```python
from build123d import *

# Parameters (mm, degrees)
SKETCH_1_R               = 17.4
EXTRUDE_1_DEPTH          = 5.6
SKETCH_2_R               = 1.7
CUT_EXTRUDE_1_DEPTH      = 26.23648153
SKETCH_3_R               = 7
CUT_EXTRUDE_2_DEPTH      = 26.23648153
SKETCH_4_R               = 2.8
CUT_EXTRUDE_3_DEPTH      = 3
SKETCH_5_R               = 1.7
CUT_EXTRUDE_4_DEPTH      = 26.23648153
CUT_EXTRUDE_5_DEPTH      = 2.5
SKETCH_7_W               = 16.1
SKETCH_7_H               = 16.1
CUT_EXTRUDE_6_DEPTH      = 1.5
CHAMFER_1_SIZE           = 0.5
SKETCH_9_W               = 2.2
SKETCH_9_H               = 8
SKETCH_9_W_2             = 8
SKETCH_9_H_2             = 2.2
CUT_EXTRUDE_7_DEPTH      = 26.281613873
BOSS_EXTRUDE1_DEPTH      = 5.6
BOSS_EXTRUDE1_DEPTH_BACK = 4
SKETCH1_R                = 20.65
SKETCH1_R_2              = 17.4
SKETCH3_R                = 23
SKETCH3_R_2              = 20.65
BOSS_EXTRUDE2_DEPTH      = 2.5
SKETCH4_R                = 18
CUT_EXTRUDE3_DEPTH       = 4
SKETCH5_W                = 1
SKETCH5_H                = 8
CUT_EXTRUDE4_DEPTH       = 10
CUT_EXTRUDE6_DEPTH       = 10
FILLET3_R                = 1
SKETCH9_R                = 23
CUT_EXTRUDE8_DEPTH       = 6.5


with BuildPart() as part:
    # 草图1 → 凸台-拉伸1 (new body)
    with BuildSketch(Plane.XY):
        Circle(SKETCH_1_R)
    extrude(amount=EXTRUDE_1_DEPTH)

    # 草图2 → 切除-拉伸1 (cut, through all)
    with BuildSketch(Plane.XY.offset(5.6)):
        with Locations((-6.717514421, 6.717514421)):
            Circle(SKETCH_2_R)
        with Locations((6.717514421, -6.717514421)):
            Circle(SKETCH_2_R)
    extrude(amount=-CUT_EXTRUDE_1_DEPTH, mode=Mode.SUBTRACT)

    # 草图3 → 切除-拉伸2 (cut, through all)
    with BuildSketch(Plane.XY.offset(5.6)):
        Circle(SKETCH_3_R)
    extrude(amount=-CUT_EXTRUDE_2_DEPTH, mode=Mode.SUBTRACT)

    # 草图4 → 切除-拉伸3 (cut)
    with BuildSketch(Plane.XY.offset(5.6)):
        with Locations((-6.717514421, 6.717514421)):
            Circle(SKETCH_4_R)
        with Locations((6.717514421, -6.717514421)):
            Circle(SKETCH_4_R)
    extrude(amount=-CUT_EXTRUDE_3_DEPTH, mode=Mode.SUBTRACT)

    # 草图5 → 切除-拉伸4 (cut, through all)
    with BuildSketch(Plane.XY.offset(5.6)):
        with Locations((8.05, 8)):
            Circle(SKETCH_5_R)
        with Locations((-8.05, -8)):
            Circle(SKETCH_5_R)
    extrude(amount=-CUT_EXTRUDE_4_DEPTH, mode=Mode.SUBTRACT)

    # 草图6 → 切除-拉伸5 (cut)
    with BuildSketch(Plane(origin=(0, 0, 0), x_dir=(-1, 0, 0), z_dir=(0, 0, -1))):
        Polygon((4.766838493, -8), (6.408419246, -10.84330127), (9.691580754, -10.84330127), (11.333161507, -8), (9.691580754, -5.15669873), (6.408419246, -5.15669873), align=None)
        Polygon((-4.766838493, 8), (-6.408419246, 10.84330127), (-9.691580754, 10.84330127), (-11.333161507, 8), (-9.691580754, 5.15669873), (-6.408419246, 5.15669873), align=None)
    extrude(amount=-CUT_EXTRUDE_5_DEPTH, mode=Mode.SUBTRACT)

    # 草图7 → 切除-拉伸6 (cut)
    with BuildSketch(Plane.XY.offset(5.6)):
        Rectangle(SKETCH_7_W, SKETCH_7_H)
    extrude(amount=-CUT_EXTRUDE_6_DEPTH, mode=Mode.SUBTRACT)

    # 倒角1
    chamfer_1_edges = [part.edges().sort_by_distance(p)[0] for p in [
        (8.05, 1.022551258, 5.6),
        (1.047918985, 8.05, 5.6),
        (-8.05, -1.022551258, 5.6),
        (-1.047918985, -8.05, 5.6),
    ]]
    chamfer(chamfer_1_edges, length=CHAMFER_1_SIZE)

    # 草图8 → 旋转1 (revolve)
    with BuildSketch(Plane(origin=(0, 0, 0), x_dir=(0, 0, -1), z_dir=(1, 0, 0)), mode=Mode.PRIVATE) as revolve_1_sk:
        Polygon((0, 17.4), (0, 17.2), (0.2, 17.4), align=None)
    revolve(revolve_1_sk.sketch.rotate(Axis((0, 0, 0), (0, 0, 1)), 90), axis=Axis((0, 0, 0), (0, 0, 1)))

    # 草图9 → 切除-拉伸7 (cut, through all)
    with BuildSketch(Plane.XY.offset(5.6)):
        with Locations((14.6, 0)):
            Rectangle(SKETCH_9_W, SKETCH_9_H)
        with Locations((0, 14.6)):
            Rectangle(SKETCH_9_W_2, SKETCH_9_H_2)
        with Locations((-14.6, 0)):
            Rectangle(SKETCH_9_W, SKETCH_9_H)
        with Locations((0, -14.6)):
            Rectangle(SKETCH_9_W_2, SKETCH_9_H_2)
    extrude(amount=-CUT_EXTRUDE_7_DEPTH, mode=Mode.SUBTRACT)

    # Sketch1 → Boss-Extrude1 (add, two sides: drawn at the far end of the back side and taken through both)
    with BuildSketch(Plane.XY.offset(-BOSS_EXTRUDE1_DEPTH_BACK)):
        Circle(SKETCH1_R)
        Circle(SKETCH1_R_2, mode=Mode.SUBTRACT)
    extrude(amount=BOSS_EXTRUDE1_DEPTH + BOSS_EXTRUDE1_DEPTH_BACK)

    # Sketch3 → Boss-Extrude2 (add)
    with BuildSketch(Plane(origin=(0, 0, -4), x_dir=(-1, 0, 0), z_dir=(0, 0, -1))):
        Circle(SKETCH3_R)
        with Locations(Location((0, 0, 0), (0, 0, 180))):
            Circle(SKETCH3_R_2, mode=Mode.SUBTRACT)
    extrude(amount=-BOSS_EXTRUDE2_DEPTH)

    # Sketch4 → Cut-Extrude3 (cut)
    with BuildSketch(Plane(origin=(0, 0, -4), x_dir=(-1, 0, 0), z_dir=(0, 0, -1))):
        Circle(SKETCH4_R)
    extrude(amount=-CUT_EXTRUDE3_DEPTH, mode=Mode.SUBTRACT)

    # Sketch5 → Cut-Extrude4 (cut)
    with BuildSketch(Plane(origin=(0, 0, -4), x_dir=(-1, 0, 0), z_dir=(0, 0, -1))):
        with Locations((22.5, 0)):
            Rectangle(SKETCH5_W, SKETCH5_H)
        with Locations((-22.5, 0)):
            Rectangle(SKETCH5_W, SKETCH5_H)
    extrude(amount=-CUT_EXTRUDE4_DEPTH, mode=Mode.SUBTRACT)

    # Sketch7 → Cut-Extrude6 (cut)
    with BuildSketch(Plane(origin=(0, 0, -4), x_dir=(-1, 0, 0), z_dir=(0, 0, -1))):
        with BuildLine():
            Line((0, 18), (0, 22.3))
            Line((0, 22.3), (-2.6, 22.3))
            Line((-2.6, 22.3), (-2.6, 17.811232411))
            ThreePointArc((-2.6, 17.811232411), (-1.303421766, 17.952746077), (0, 18))
        make_face()
        with BuildLine():
            Line((0, 17.5), (0, 18))
            ThreePointArc((0, 18), (-1.303421766, 17.952746077), (-2.6, 17.811232411))
            Line((-2.6, 17.811232411), (-2.6, 17.5))
            Line((-2.6, 17.5), (0, 17.5))
        make_face()
        with BuildLine():
            Line((2.6, 22.3), (0, 22.3))
            Line((0, 22.3), (0, 18))
            ThreePointArc((0, 18), (1.303421766, 17.952746077), (2.6, 17.811232411))
            Line((2.6, 17.811232411), (2.6, 22.3))
        make_face()
        with BuildLine():
            ThreePointArc((2.6, 17.811232411), (1.303421766, 17.952746077), (0, 18))
            Line((0, 18), (0, 17.5))
            Line((0, 17.5), (2.6, 17.5))
            Line((2.6, 17.5), (2.6, 17.811232411))
        make_face()
    extrude(amount=-CUT_EXTRUDE6_DEPTH, mode=Mode.SUBTRACT)

    # Fillet3
    # the kernel refuses this fillet: 1 mm, written as the material it adds along each edge
    with BuildSketch(Plane(origin=(2.6, 22.3, -4), x_dir=(-1, 0, 0), z_dir=(0, 0, 1))) as fillet3_piece_1:
        with BuildLine():
            CenterArc((FILLET3_R, FILLET3_R), FILLET3_R, 180, 90)
            Line((0, FILLET3_R), (-FILLET3_R * 0.02, FILLET3_R))
            Line((-FILLET3_R * 0.02, FILLET3_R), (-FILLET3_R * 0.02, -FILLET3_R * 0.02))
            Line((-FILLET3_R * 0.02, -FILLET3_R * 0.02), (FILLET3_R, -FILLET3_R * 0.02))
            Line((FILLET3_R, -FILLET3_R * 0.02), (FILLET3_R, 0))
        make_face()
    extrude(amount=2.5)
    with BuildSketch(Plane(origin=(-2.6, 22.3, -4), x_dir=(1, 0, 0), z_dir=(0, 0, 1))) as fillet3_piece_2:
        with BuildLine():
            CenterArc((FILLET3_R, -FILLET3_R), FILLET3_R, 90, 90)
            Line((0, -FILLET3_R), (-FILLET3_R * 0.02, -FILLET3_R))
            Line((-FILLET3_R * 0.02, -FILLET3_R), (-FILLET3_R * 0.02, FILLET3_R * 0.02))
            Line((-FILLET3_R * 0.02, FILLET3_R * 0.02), (FILLET3_R, FILLET3_R * 0.02))
            Line((FILLET3_R, FILLET3_R * 0.02), (FILLET3_R, 0))
        make_face()
    extrude(amount=2.5)
    with BuildSketch(Plane(origin=(-2.6, 17.5, -6), x_dir=(0, 1, 0), z_dir=(0, 0, 1))) as fillet3_piece_3_section:
        with BuildLine():
            CenterArc((FILLET3_R, -FILLET3_R), FILLET3_R, 90, 90)
            Line((0, -FILLET3_R), (-FILLET3_R * 0.02, -FILLET3_R))
            Line((-FILLET3_R * 0.02, -FILLET3_R), (-FILLET3_R * 0.02, FILLET3_R * 0.02))
            Line((-FILLET3_R * 0.02, FILLET3_R * 0.02), (FILLET3_R, FILLET3_R * 0.02))
            Line((FILLET3_R, FILLET3_R * 0.02), (FILLET3_R, 0))
        make_face()
    fillet3_piece_3 = extrude(amount=11.6, mode=Mode.PRIVATE)
    fillet3_piece_3 = split(fillet3_piece_3, bisect_by=Plane(origin=(-2.544482942, 18.024809788, 0), z_dir=(0, 0, -1)), keep=Keep.TOP, mode=Mode.PRIVATE)
    fillet3_piece_3 = fillet3_piece_3 - Plane(origin=(0, 0, -2), x_dir=(-1, 0, 0), z_dir=(0, 0, -1)) * Cylinder(18, 28, mode=Mode.PRIVATE)
    fillet3_piece_3 = split(fillet3_piece_3, bisect_by=Plane(origin=(-2.544482942, 18.024809788, -4), z_dir=(0, 0, 1)), keep=Keep.TOP, mode=Mode.PRIVATE)
    add(fillet3_piece_3)
    with BuildSketch(Plane(origin=(-2.6, 17.5, 0), x_dir=(0, 1, 0), z_dir=(0, 0, 1))) as fillet3_piece_4_section:
        with BuildLine():
            CenterArc((FILLET3_R, -FILLET3_R), FILLET3_R, 90, 90)
            Line((0, -FILLET3_R), (-FILLET3_R * 0.02, -FILLET3_R))
            Line((-FILLET3_R * 0.02, -FILLET3_R), (-FILLET3_R * 0.02, FILLET3_R * 0.02))
            Line((-FILLET3_R * 0.02, FILLET3_R * 0.02), (FILLET3_R, FILLET3_R * 0.02))
            Line((FILLET3_R, FILLET3_R * 0.02), (FILLET3_R, 0))
        make_face()
    fillet3_piece_4 = extrude(amount=5.6, mode=Mode.PRIVATE)
    fillet3_piece_4 = fillet3_piece_4 - Plane(origin=(0, 0, 2.8), x_dir=(-1, 0, 0), z_dir=(0, 0, -1)) * Cylinder(18, 16, mode=Mode.PRIVATE)
    add(fillet3_piece_4)
    with BuildSketch(Plane(origin=(-2.6, 17.5, 0), x_dir=(0, 1, 0), z_dir=(0, 0, 1))) as fillet3_piece_5_section:
        with BuildLine():
            CenterArc((FILLET3_R, -FILLET3_R), FILLET3_R, 90, 90)
            Line((0, -FILLET3_R), (-FILLET3_R * 0.02, -FILLET3_R))
            Line((-FILLET3_R * 0.02, -FILLET3_R), (-FILLET3_R * 0.02, FILLET3_R * 0.02))
            Line((-FILLET3_R * 0.02, FILLET3_R * 0.02), (FILLET3_R, FILLET3_R * 0.02))
            Line((FILLET3_R, FILLET3_R * 0.02), (FILLET3_R, 0))
        make_face()
    fillet3_piece_5 = extrude(amount=5.6, mode=Mode.PRIVATE)
    fillet3_piece_5 = fillet3_piece_5 & Plane(origin=(0, 0, 2.8), x_dir=(-1, 0, 0), z_dir=(0, 0, -1)) * Cylinder(18, 16, mode=Mode.PRIVATE)
    add(fillet3_piece_5)
    with BuildSketch(Plane(origin=(2.6, 17.5, -6), x_dir=(-1, 0, 0), z_dir=(0, 0, 1))) as fillet3_piece_6_section:
        with BuildLine():
            CenterArc((FILLET3_R, -FILLET3_R), FILLET3_R, 90, 90)
            Line((0, -FILLET3_R), (-FILLET3_R * 0.02, -FILLET3_R))
            Line((-FILLET3_R * 0.02, -FILLET3_R), (-FILLET3_R * 0.02, FILLET3_R * 0.02))
            Line((-FILLET3_R * 0.02, FILLET3_R * 0.02), (FILLET3_R, FILLET3_R * 0.02))
            Line((FILLET3_R, FILLET3_R * 0.02), (FILLET3_R, 0))
        make_face()
    fillet3_piece_6 = extrude(amount=11.6, mode=Mode.PRIVATE)
    fillet3_piece_6 = split(fillet3_piece_6, bisect_by=Plane(origin=(2.544482942, 18.024809788, 0), z_dir=(0, 0, -1)), keep=Keep.TOP, mode=Mode.PRIVATE)
    fillet3_piece_6 = fillet3_piece_6 - Plane(origin=(0, 0, -2), x_dir=(-1, 0, 0), z_dir=(0, 0, -1)) * Cylinder(18, 28, mode=Mode.PRIVATE)
    fillet3_piece_6 = split(fillet3_piece_6, bisect_by=Plane(origin=(2.544482942, 18.024809788, -4), z_dir=(0, 0, 1)), keep=Keep.TOP, mode=Mode.PRIVATE)
    add(fillet3_piece_6)
    with BuildSketch(Plane(origin=(2.6, 17.5, 0), x_dir=(-1, 0, 0), z_dir=(0, 0, 1))) as fillet3_piece_7_section:
        with BuildLine():
            CenterArc((FILLET3_R, -FILLET3_R), FILLET3_R, 90, 90)
            Line((0, -FILLET3_R), (-FILLET3_R * 0.02, -FILLET3_R))
            Line((-FILLET3_R * 0.02, -FILLET3_R), (-FILLET3_R * 0.02, FILLET3_R * 0.02))
            Line((-FILLET3_R * 0.02, FILLET3_R * 0.02), (FILLET3_R, FILLET3_R * 0.02))
            Line((FILLET3_R, FILLET3_R * 0.02), (FILLET3_R, 0))
        make_face()
    fillet3_piece_7 = extrude(amount=5.6, mode=Mode.PRIVATE)
    fillet3_piece_7 = fillet3_piece_7 & Plane(origin=(0, 0, 2.8), x_dir=(-1, 0, 0), z_dir=(0, 0, -1)) * Cylinder(18, 16, mode=Mode.PRIVATE)
    add(fillet3_piece_7)
    with BuildSketch(Plane(origin=(2.6, 17.5, 0), x_dir=(-1, 0, 0), z_dir=(0, 0, 1))) as fillet3_piece_8_section:
        with BuildLine():
            CenterArc((FILLET3_R, -FILLET3_R), FILLET3_R, 90, 90)
            Line((0, -FILLET3_R), (-FILLET3_R * 0.02, -FILLET3_R))
            Line((-FILLET3_R * 0.02, -FILLET3_R), (-FILLET3_R * 0.02, FILLET3_R * 0.02))
            Line((-FILLET3_R * 0.02, FILLET3_R * 0.02), (FILLET3_R, FILLET3_R * 0.02))
            Line((FILLET3_R, FILLET3_R * 0.02), (FILLET3_R, 0))
        make_face()
    fillet3_piece_8 = extrude(amount=5.6, mode=Mode.PRIVATE)
    fillet3_piece_8 = fillet3_piece_8 - Plane(origin=(0, 0, 2.8), x_dir=(-1, 0, 0), z_dir=(0, 0, -1)) * Cylinder(18, 16, mode=Mode.PRIVATE)
    add(fillet3_piece_8)

    # Sketch9 → Cut-Extrude8 (cut)
    with BuildSketch(Plane(origin=(0, 0, -4), x_dir=(-1, 0, 0), z_dir=(0, 0, -1))):
        Circle(SKETCH9_R)
    extrude(amount=-CUT_EXTRUDE8_DEPTH, mode=Mode.SUBTRACT)


solid = part.part
```
Design review of the part built by this model. Coordinates are the model's own, in mm. A direction names the side the tool comes from. Round coordinates to 2 decimals unless told otherwise and drop trailing zeros. Order: outer loops, then holes, each group sorted by start corner. A loop starts at its lowest first (then second) coordinate and runs counter-clockwise, first axis right, second up. Notation, with made-up numbers: (-18, -30) - (-11, -30) arc R4 cw to (-11, -26) - close; hole circle Ø2 at (41, 35). An arc over 180 degrees is marked (long way). Return JSON: item names as keys, results as strings.
Q1. The part is to be moulded in two halves that separate along Y. For faces 1 (the cylindrical face through (-2.315, 17.801, 4.028)), 2 (the flat face through (-6, -5, 4.1)), 3 (the flat face through (-9, 0, 2.5)), 4 (the flat face through (-4, -15, 4)), say which applies: pulls with the +Y half, pulls with the -Y half, needs draft (parallel to the pull), parting line crosses it, or undercut.
Computed values:
{"face 1": "pulls with the +Y half", "face 2": "undercut", "face 3": "needs draft", "face 4": "undercut"}
Q2. Wall thickness on L1, parallel to X at y = 0, z = 3.5; L2, parallel to Y at x = -2.5, z = 4.15; L3, parallel to X at y = -9, z = 3.8: over which ranges is each line inside the solid? List them lowest first. Write a range as [from, to].
Computed values:
{"L1": "x = [-20.65, -15.7], [-13.5, -7], [7, 13.5], [15.7, 20.65]", "L2": "y = [-20.5, -15.7], [-13.5, -8.05], [8.05, 13.5], [15.7, 18.06]", "L3": "x = [-18.59, -9.42], [-6.68, 5.1], [8.34, 18.59]"}
Q3. Consider section A-A on y = 0. Write out the cut boundary in (x, z).
Computed values:
{"outline": "(-20.65, 2.5) - (-15.7, 2.5) - (-15.7, 5.6) - (-20.65, 5.6) - close; (-13.5, 2.5) - (-7, 2.5) - (-7, 4.1) - (-8.05, 4.1) - (-8.05, 5.1) - (-8.55, 5.6) - (-13.5, 5.6) - close; (7, 2.5) - (13.5, 2.5) - (13.5, 5.6) - (8.55, 5.6) - (8.05, 5.1) - (8.05, 4.1) - (7, 4.1) - close; (15.7, 2.5) - (20.65, 2.5) - (20.65, 5.6) - (15.7, 5.6) - close"}
Q4. For pin 1 Ø1.8 at (x, z) = (-14.5, 3.5) entering from +Y; pin 2 Ø10 at (x, y) = (-0.5, -3) entering from +Z; pin 3 Ø1.8 at (y, z) = (-14.5, 4) entering from +X, all flat-tipped, find the tip position at first contact; note any pin that passes through.
Computed values:
{"pin 1": "stops at y = 15.54", "pin 2": "stops at z = 4.1", "pin 3": "stops at x = 15.54"}
Q5. Consider section C-C on y = -13. Write out the cut boundary in (x, z).
Computed values:
{"outline": "(-16.04, 2.5) - (16.04, 2.5) - (16.04, 5.6) - (-16.04, 5.6) - close"}
Q6. Machinability: for faces 5 (the flat face through (0, 17.5, 4)), 6 (the flat face through (-13.5, 0, 4)), 7 (the cylindrical face through (-8.62, 8.77, 3.79)), which of the approach directions +Z, -Z, +X, -X, +Y, -Y give a long, thin tool a straight path to every point of the face, cutting with its end or side? Answer none if there is none.
Computed values:
{"face 5": "+Z, -Z, +Y", "face 6": "+Z, -Z", "face 7": "+Z"}
Q7. Consider section B-B on z = 3.15. Write out the cut boundary in (x, y).
Computed values:
{"outline": "(-2.6, 18.5) - (-2.6, 20.49) arc R20.65 ccw (long way) to (2.6, 20.49) - (2.6, 18.5) arc R1 cw to (1.6, 17.5) - (-1.6, 17.5) arc R1 cw to start; hole (-15.7, -4) - (-13.5, -4) - (-13.5, 4) - (-15.7, 4) - close; hole circle Ø3.4 at (-8.05, -8); hole (-5.65, 4.13) arc R7 ccw to (4.13, -5.65) arc R2.8 ccw (long way) to (5.65, -4.13) arc R7 ccw to (-4.13, 5.65) arc R2.8 ccw (long way) to start; hole (-4, -15.7) - (4, -15.7) - (4, -13.5) - (-4, -13.5) - close; hole (-4, 13.5) - (4, 13.5) - (4, 15.7) - (-4, 15.7) - close; hole circle Ø3.4 at (8.05, 8); hole (13.5, -4) - (15.7, -4) - (15.7, 4) - (13.5, 4) - close"}
